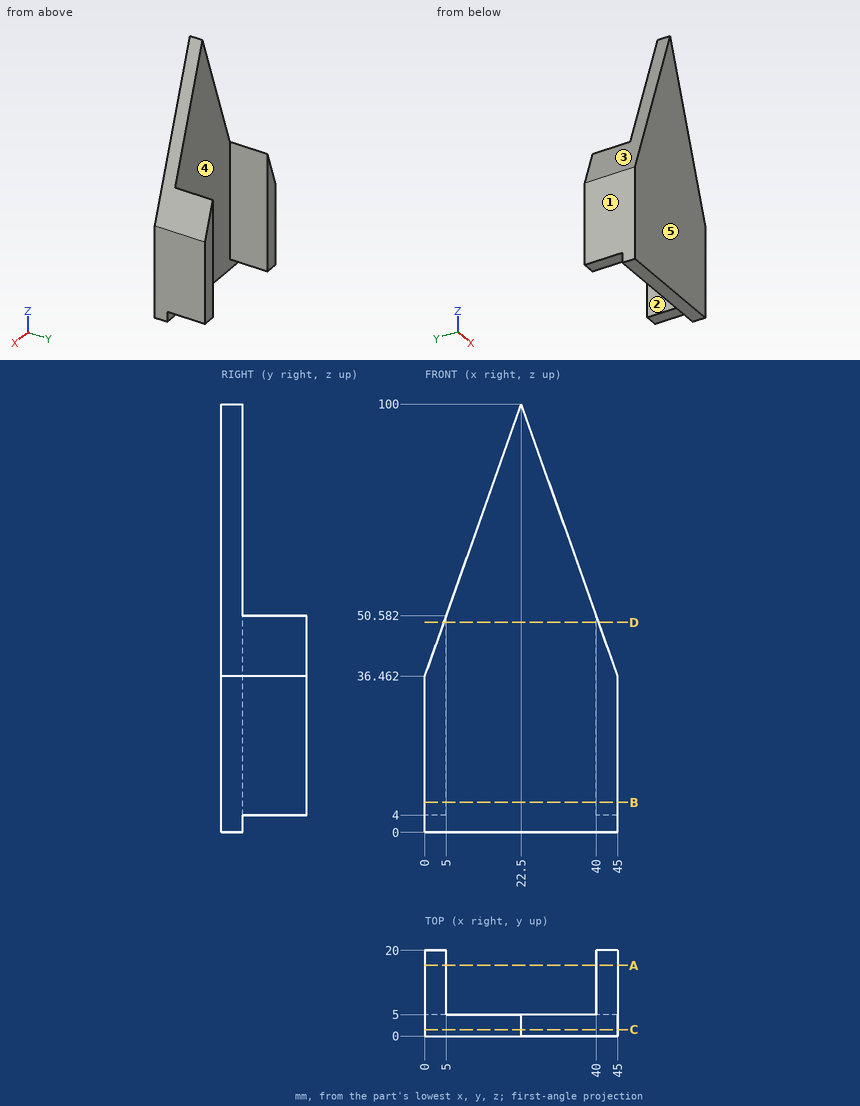
Input: dimensioned drawing with shaded views. Units: mm. Origin: part minimum x, y, z. A direction names the side the tool comes from. Round coordinates to 2 decimals unless told otherwise and drop trailing zeros. Write each loop counter-clockwise with the first axis right and the second up, starting at its lowest first coordinate (ties: lowest second). Pieces come first, ordered by that corner, then holes. Notation, with made-up numbers: (61.5, 10) -> (110.5, 10) arc R28 ccw to (110.5, 30) -> close; hole circle Ø11 at (33, 60). An arc over 180 degrees is marked (long way). Use CSV: the item, a comma, the result in double quotes. Start each with the question number.
Q1. Section A-A (y = 16.5). Return loops of the section in (x, z).
Q2. First-contact query: pin 1 Ø8 at (x, z) = (11, 58) entering from +Y; pin 2 Ø4 at (x, y) = (43.5, 12.5) entering from -Z; pin 3 Ø3 at (y, z) = (12, 48) entering from -X (1 decimal). Flat tips, straight axial feed; report the tip coordinate or a pass-through.
Q3. Line query: L1, parallel to X at y = 17, z = 29; L2, parallel to X at y = 15.5, z = 48 (1 decimal); L3, parallel to Y at x = 24.5, z = 63.5. Output: solid intervals per line, ascending.
Q4. Reachability of the marked faces 1 and 2 from +Z, -Z, +X, -X, +Y, -Y: full face, straight path, thin tool, end or side. Return the list, or none.
Q5. Section C-C (y = 1.5). Return loops of the section in (x, z), plus the area to 3 significant figures.
Q6. Section B-B (z = 7). Return loops of the section in (x, y), plus the area to 3 significant figures.
Q7. Section D-D (z = 49). Return loops of the section in (x, y).
Q8. Pull-direction query (X, two-part tool) for the marked faces 3, 4 and 5; classes: pulls with the +X half, pulls with the -X half, needs draft (parallel to the pull), parting line crosses it, or undercut.
Result sheet:
1,outline,"(0, 4) -> (5, 4) -> (5, 50.58) -> (0, 36.46) -> close; (40, 4) -> (45, 4) -> (45, 36.46) -> (40, 50.58) -> close"
2,pin 1,"y = 5"
2,pin 2,"z = 4"
2,pin 3,"x = 3.6"
3,L1,"0 to 5, 40 to 45"
3,L2,"4.1 to 5, 40 to 40.9"
3,L3,"0 to 5"
4,face 1,"+Z, -Z, -X, +Y, -Y"
4,face 2,"+Z, -Z, +Y"
5,outline,"(0, 0) -> (45, 0) -> (45, 36.46) -> (22.5, 100) -> (0, 36.46) -> close"
5,area,"3,070 mm²"
6,outline,"(0, 0) -> (45, 0) -> (45, 20) -> (40, 20) -> (40, 5) -> (5, 5) -> (5, 20) -> (0, 20) -> close"
6,area,"375 mm²"
7,outline,"(4.44, 0) -> (40.56, 0) -> (40.56, 20) -> (40, 20) -> (40, 5) -> (5, 5) -> (5, 20) -> (4.44, 20) -> close"
8,face 3,"pulls with the -X half"
8,face 4,"undercut"
8,face 5,"needs draft"
